Read the model definition and answer for the solid it produces. Units are mm, in the model's axes. Give positions to 0.01 mm unless a question says otherwise; leave off trailing zeros. Loops run counter-clockwise (first coordinate to the right, second up) from the corner with the lowest first, then second, coordinate; pieces in that order, holes last.
(1) Find section C-C, the plane z = 4. State how many separate pieces and enclosed holes the cut face has, then the cut area to 3 significant figures.
(2) Each of these flat-tipped pins is pushed along its axis until it touches: P1, Ø1.5, axis at y = -3.5, z = 4, coming from the +X side; P2, Ø2, axis at y = 96.5, z = 4, coming from the -X side. Where does it stop, or does it pass through?
(3) Find section B-B, the plane x = 55. Write down the section's boundary in (y, z), then the cut area to 3 significant figures.
(4) Find section A-A, the plane y = 14.5. Write down the section's boundary in (x, z), then the cut area to 3 significant figures.
(5) Straight lines are drawn through the part: probe 1 along X at (y, z) = (-8.5, 5); probe 2 along Y at (x, z) = (10.5, 9); probe 3 along Y at (x, z) = (-4.5, 8.75). For each, find the intervals that lie inside material, in ascending order.
```python
from build123d import *

# Parameters (mm, degrees)
SKETCH1_W           = 40.5
SKETCH1_H           = 81
BOSS_EXTRUDE1_DEPTH = 10
FILLET1_R           = 3


with BuildPart() as part:
    # Sketch1 → Boss-Extrude1 (new body)
    with BuildSketch(Plane.XY):
        Polygon((-64, 129.5), (-64, 125.5), (-47, 125.5), (-47, 44.5), (-64, 44.5), (-64, 40.5), (-47, 40.5), (-47, -40.5), (-64, -40.5), (-64, -44.5), (0, -44.5), (64, -44.5), (64, -40.5), (47, -40.5), (47, 40.5), (64, 40.5), (64, 44.5), (47, 44.5), (47, 125.5), (64, 125.5), (64, 129.5), (0, 129.5), align=None)
        with Locations((-22.75, 0)):
            Rectangle(SKETCH1_W, SKETCH1_H, mode=Mode.SUBTRACT)
        with Locations((22.75, 0)):
            Rectangle(SKETCH1_W, SKETCH1_H, mode=Mode.SUBTRACT)
        with Locations((-22.75, 85)):
            Rectangle(SKETCH1_W, SKETCH1_H, mode=Mode.SUBTRACT)
        with Locations((22.75, 85)):
            Rectangle(SKETCH1_W, SKETCH1_H, mode=Mode.SUBTRACT)
    extrude(amount=BOSS_EXTRUDE1_DEPTH)

    # Fillet1
    fillet1_edges = [part.edges().sort_by_distance(p)[0] for p in [
        (43, -40.5, 5),
        (43, 40.5, 5),
        (2.5, 40.5, 5),
        (2.5, -40.5, 5),
        (43, 44.5, 5),
        (43, 125.5, 5),
        (2.5, 125.5, 5),
        (2.5, 44.5, 5),
        (-43, 40.5, 5),
        (-43, -40.5, 5),
        (-2.5, -40.5, 5),
        (-2.5, 40.5, 5),
        (-43, 125.5, 5),
        (-43, 44.5, 5),
        (-2.5, 44.5, 5),
        (-2.5, 125.5, 5),
        (-47, 44.5, 5),
        (-47, 125.5, 5),
        (47, 125.5, 5),
        (47, 44.5, 5),
        (47, 40.5, 5),
        (47, -40.5, 5),
        (-47, -40.5, 5),
        (-47, 40.5, 5),
    ]]
    fillet(fillet1_edges, radius=FILLET1_R)


solid = part.part
```
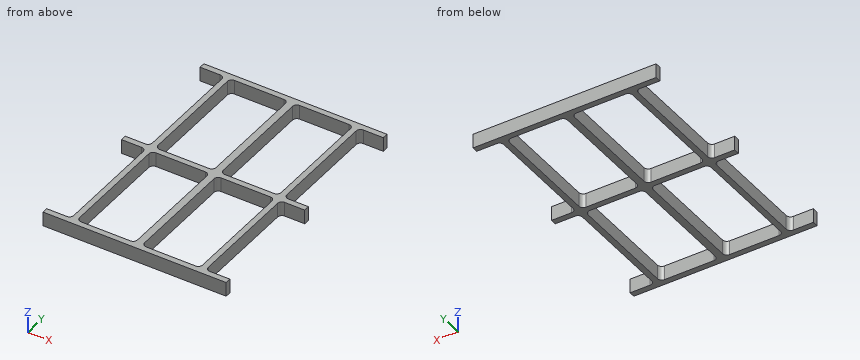
Entries:
1. separate pieces: 1
1. enclosed holes: 4
1. area: 3,690 mm2
2. P1: stops at x = 47
2. P2: stops at x = -47
3. outline: (-44.5, 0) - (-40.5, 0) - (-40.5, 10) - (-44.5, 10) - close; (40.5, 0) - (44.5, 0) - (44.5, 10) - (40.5, 10) - close; (125.5, 0) - (129.5, 0) - (129.5, 10) - (125.5, 10) - close
3. area: 120 mm2
4. outline: (-47, 0) - (-43, 0) - (-43, 10) - (-47, 10) - close; (-2.5, 0) - (2.5, 0) - (2.5, 10) - (-2.5, 10) - close; (43, 0) - (47, 0) - (47, 10) - (43, 10) - close
4. area: 130 mm2
5. probe 1: x = -47 to -43, -2.5 to 2.5, 43 to 47
5. probe 2: y = -44.5 to -40.5, 40.5 to 44.5, 125.5 to 129.5
5. probe 3: y = -44.5 to -40.33, 40.33 to 44.67, 125.33 to 129.5
